The model under review builds one solid part; all positions refer to its coordinate system, in mm. A direction names the side the tool comes from. Round coordinates to 2 decimals unless told otherwise and drop trailing zeros. Loops run counter-clockwise (first coordinate to the right, second up) from the corner with the lowest first, then second, coordinate; pieces in that order, holes last. Notation, with made-up numbers: M -9,33.25 L 33,33.25 A22 cw 33,50.25 Z; hole C 77,33 d2. An arc over 180 degrees is marked long. Return JSON: item names as keys, results as strings. Group by question number.
Q1. To check wall thickness, follow line 1 along Y through (x, z) = (0, 3); line 2 along Y through (x, z) = (4.5, 9.5); line 3 along X through (y, z) = (36, 1.5). State the ranges of each line that lie inside material, in increasing order.
Q2. Consider section A-A (z = 4.75). State the section outline as (x, y) points.
Q3. Draft analysis for pull direction Y (two halves, no side actions). For faces 4 (the face through (-9.538, -42.954, 4.93)), 5 (the face through (-27, 0, 6)), 6 (the face through (40, 0, 1)), 7 (the face through (-10.4, 20.2, 0)), state which applies: pulls with the +Y half, pulls with the -Y half, needs draft (parallel to the pull), parting line crosses it, or undercut.
Q4. Consider section D-D (y = 0). State the section outline as (x, z) points.
Q5. Consider section C-C (y = -37). State the section outline as (x, z) points, and give its area (3 significant figures).
Q6. Clearance check with flat-ended pins moving along their axes: pin 1 Ø12 at (x, y) = (-8.5, -13.5) entering from -Z; pin 2 Ø2 at (x, z) = (-30, 6.5) entering from +Y; pin 3 Ø4 at (y, z) = (-7.5, 3) entering from -X; pin 4 Ø7.5 at (x, y) = (-3.5, 34.5) entering from +Z. State where each tip first meets the part, or that it passes through.
Q7. Consider section B-B (x = 32.5). State the section outline as (y, z) points.
Q8. For faces 1 (the face through (-8, -35, 6)), 2 (the face through (-20.2, 10.4, 10)), 3 (the face through (-40, 0, 1)), list the 3-axis set-ups (+Z, -Z, +X, -X, +Y, -Y) from which the entire face can be reached by the end or side of a thin tool; tool diameter is ignored.
from build123d import *

# Parameters (mm, degrees)
IZIM1_R                                     = 44
IZIM1_R_2                                   = 22.5
Y_KSEKLIK_EKSTR_ZYON1_DEPTH                 = 10
M8_START                                    = 1.4
M8_ALT_GEN_ALYAN_BA_L_K_R_VIDA_IN_HAV_DEPTH = 8.6
M8_ALT_GEN_ALYAN_BA_L_K_R_VIDA_IN_3_DEPTH   = 1.4


# Read off the part's stored shape, not the designer's step: M8 Altıgen Alyan Başlı Kör Vida İçin Havşa1
with BuildPart() as part:
    # Çizim1 → Yükseklik-Ekstrüzyon1 (new body)
    with BuildSketch(Plane.XY):
        Circle(IZIM1_R)
        Circle(IZIM1_R_2, mode=Mode.SUBTRACT)
    extrude(amount=Y_KSEKLIK_EKSTR_ZYON1_DEPTH)

    # M8 Alt_gen Alyan Ba_l_ K_r Vida _in  2 → M8 Altıgen Alyan Başlı Kör Vida İçin Havşa1 (cut)
    with BuildSketch(Plane.XY.offset(M8_START)):
        with BuildLine():
            Line((-35.031641101, -7.516581593), (-34.033584774, -7.454263318))
            ThreePointArc((-34.033584774, -7.454263318), (-27.015549381, 0.4985462), (-34.968358899, 7.516581593))
            Line((-34.968358899, 7.516581593), (-35.966415226, 7.454263318))
            ThreePointArc((-35.966415226, 7.454263318), (-42.984450619, -0.4985462), (-35.031641101, -7.516581593))
        make_face()
        with BuildLine():
            Line((-0.031641101, -42.516581593), (0.966415226, -42.454263318))
            ThreePointArc((0.966415226, -42.454263318), (7.984450619, -34.5014538), (0.031641101, -27.483418407))
            Line((0.031641101, -27.483418407), (-0.966415226, -27.545736682))
            ThreePointArc((-0.966415226, -27.545736682), (-7.984450619, -35.4985462), (-0.031641101, -42.516581593))
        make_face()
        with BuildLine():
            Line((34.968358899, -7.516581593), (35.966415226, -7.454263318))
            ThreePointArc((35.966415226, -7.454263318), (42.984450619, 0.4985462), (35.031641101, 7.516581593))
            Line((35.031641101, 7.516581593), (34.033584774, 7.454263318))
            ThreePointArc((34.033584774, 7.454263318), (27.015549381, -0.4985462), (34.968358899, -7.516581593))
        make_face()
        with BuildLine():
            Line((-0.031641101, 27.483418407), (0.966415226, 27.545736682))
            ThreePointArc((0.966415226, 27.545736682), (7.984450619, 35.4985462), (0.031641101, 42.516581593))
            Line((0.031641101, 42.516581593), (-0.966415226, 42.454263318))
            ThreePointArc((-0.966415226, 42.454263318), (-7.984450619, 34.5014538), (-0.031641101, 27.483418407))
        make_face()
    extrude(amount=M8_ALT_GEN_ALYAN_BA_L_K_R_VIDA_IN_HAV_DEPTH, mode=Mode.SUBTRACT)

    # M8 Alt_gen Alyan Ba_l_ K_r Vida _in 3 ou → M8 Alt_gen Alyan Ba_l_ K_r Vida _in  3 (cut)
    with BuildSketch(Plane.XY):
        with BuildLine():
            Line((-35.218595926, -4.522412611), (-34.220539599, -4.460094336))
            ThreePointArc((-34.220539599, -4.460094336), (-30.009718363, 0.311591375), (-34.781404074, 4.522412611))
            Line((-34.781404074, 4.522412611), (-35.779460401, 4.460094336))
            ThreePointArc((-35.779460401, 4.460094336), (-39.990281637, -0.311591375), (-35.218595926, -4.522412611))
        make_face()
        with BuildLine():
            ThreePointArc((-0.779460401, -30.539905664), (-4.990281637, -35.311591375), (-0.218595926, -39.522412611))
            Line((-0.218595926, -39.522412611), (0.779460401, -39.460094336))
            ThreePointArc((0.779460401, -39.460094336), (4.990281637, -34.688408625), (0.218595926, -30.477587389))
            Line((0.218595926, -30.477587389), (-0.779460401, -30.539905664))
        make_face()
        with BuildLine():
            Line((34.781404074, -4.522412611), (35.779460401, -4.460094336))
            ThreePointArc((35.779460401, -4.460094336), (39.990281637, 0.311591375), (35.218595926, 4.522412611))
            Line((35.218595926, 4.522412611), (34.220539599, 4.460094336))
            ThreePointArc((34.220539599, 4.460094336), (30.009718363, -0.311591375), (34.781404074, -4.522412611))
        make_face()
        with BuildLine():
            ThreePointArc((0.779460401, 30.539905664), (4.990281637, 35.311591375), (0.218595926, 39.522412611))
            Line((0.218595926, 39.522412611), (-0.779460401, 39.460094336))
            ThreePointArc((-0.779460401, 39.460094336), (-4.990281637, 34.688408625), (-0.218595926, 30.477587389))
            Line((-0.218595926, 30.477587389), (0.779460401, 30.539905664))
        make_face()
    extrude(amount=M8_ALT_GEN_ALYAN_BA_L_K_R_VIDA_IN_3_DEPTH, mode=Mode.SUBTRACT)


solid = part.part
Values:
{
 "1": {"line 1": "y = -44 to -42.51, -27.49 to -22.5, 22.5 to 27.49, 42.51 to 44", "line 2": "y = -43.77 to -41.31, -28.63 to -22.05, 22.05 to 28.69, 41.37 to 43.77", "line 3": "x = -25.3 to -7.93, 7.94 to 25.3"},
 "2": {"outline": "C 0,0 d88; hole M -35.97,7.45 A7.5 ccw -35.03,-7.52 L -34.03,-7.45 A7.5 ccw -34.97,7.52 Z; hole C 0,0 d45; hole M -0.97,-27.55 A7.5 ccw -0.03,-42.52 L 0.97,-42.45 A7.5 ccw 0.03,-27.48 Z; hole M -0.97,42.45 A7.5 ccw -0.03,27.48 L 0.97,27.55 A7.5 ccw 0.03,42.52 Z; hole M 34.03,7.45 A7.5 ccw 34.97,-7.52 L 35.97,-7.45 A7.5 ccw 35.03,7.52 Z"},
 "3": {"face 4": "parting line crosses it", "face 5": "undercut", "face 6": "undercut", "face 7": "needs draft"},
 "4": {"outline": "M -44,0 L -40,0 L -40,1.4 L -43,1.4 L -43,10 L -44,10 Z; M -30,0 L -22.5,0 L -22.5,10 L -27,10 L -27,1.4 L -30,1.4 Z; M 22.5,0 L 30,0 L 30,1.4 L 27,1.4 L 27,10 L 22.5,10 Z; M 40,0 L 44,0 L 44,10 L 43,10 L 43,1.4 L 40,1.4 Z"},
 "5": {"outline": "M -23.81,0 L -4.55,0 L -4.55,1.4 L -7.74,1.4 L -7.74,10 L -23.81,10 Z; M 4.51,0 L 23.81,0 L 23.81,10 L 7.72,10 L 7.72,1.4 L 4.51,1.4 Z", "area": "331 mm2"},
 "6": {"pin 1": "passes through", "pin 2": "stops at y = 33.09", "pin 3": "stops at x = -43.65", "pin 4": "stops at z = 1.4"},
 "7": {"outline": "M -29.66,0 L -4.06,0 L -4.06,1.4 L -7.26,1.4 L -7.26,10 L -29.66,10 Z; M 4,0 L 29.66,0 L 29.66,10 L 7.2,10 L 7.2,1.4 L 4,1.4 Z"},
 "8": {"face 1": "+Z", "face 2": "+Z, +X, -X, +Y, -Y", "face 3": "+Z, -Z"}
}
